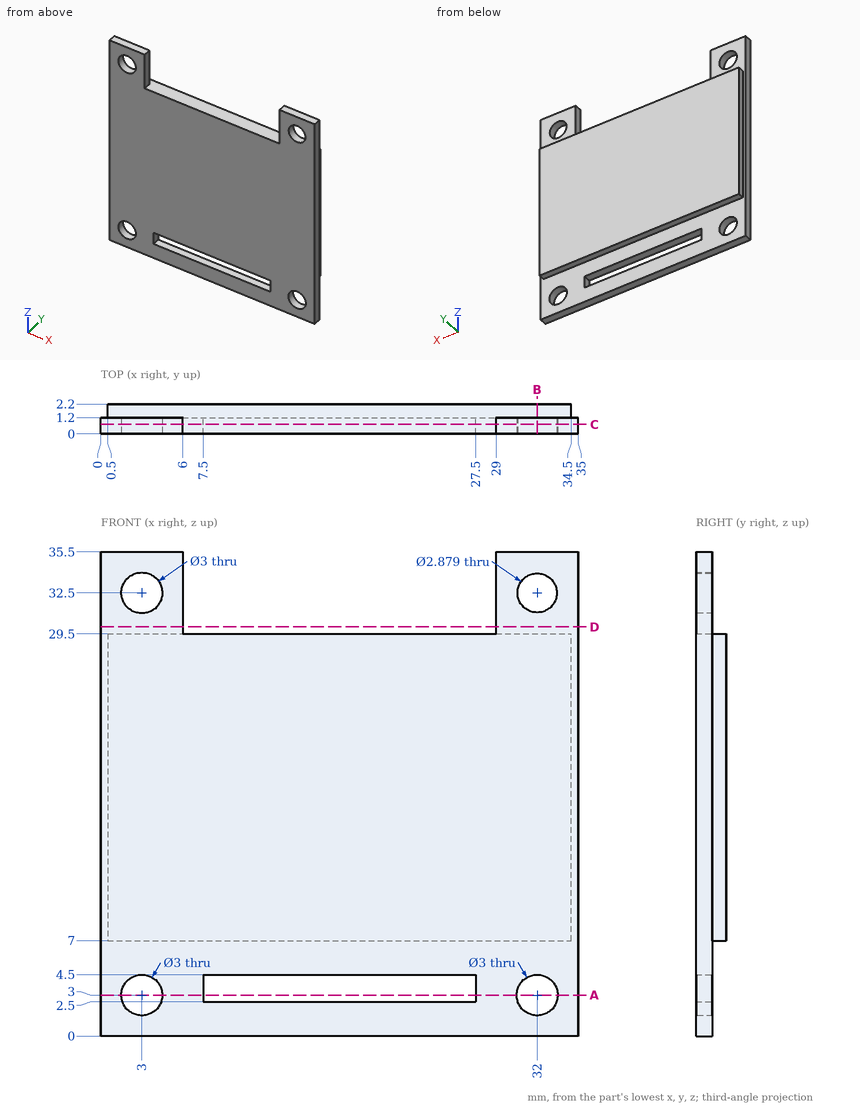
Check sheet for the drawn part. Datum: minimum x, y, z corner. Units: mm. Give positions to 0.01 mm unless a question says otherwise; leave off trailing zeros. Write each loop counter-clockwise with the first axis right and the second up, starting at its lowest first coordinate (ties: lowest second). Pieces come first, ordered by that corner, then holes. Notation, with made-up numbers: (79.5, -22) -> (85.5, -22) arc R36 ccw to (85.5, 12) -> close; hole circle Ø10 at (-39, 81.5). An arc over 180 degrees is marked (long way). Use one line per item in the form item = value. Start each with the question number.
1. Go/stop test with flat-tipped pins: P1, Ø0.8, axis at x = 20, y = 2, coming from the -Z side; P2, Ø1, axis at x = 13.5, y = 0.5, coming from the -Z side; P3, Ø3.5, axis at x = 3, z = 32.5, coming from the +Y side; P4, Ø2.5, axis at x = 32, z = 32.5, coming from the -Y side. Record where each tip stops, or that it passes through.
2. Section check D-D (z = 30). Record the cut outline in (x, y), and give its area (3 significant figures).
3. Section check C-C (y = 0.7). Record the cut outline in (x, z).
4. Section check B-B (x = 32). Record the cut outline in (y, z).
5. Section check A-A (z = 3). Record the cut outline in (x, y), and give its area (3 significant figures).
6. Thickness scan on line 1 along X through (y, z) = (0.7, 32.5); line 2 along X through (y, z) = (0.65, 3); line 3 along Z through (x, y) = (31, 0.9) (1 decimal). Record the ranges inside material, lowest first. Write a range as from..to.
Conclusion:
q1.P1 = 7
q1.P2 = 0
q1.P3 = 1.2
q1.P4 = through
q2.outline = (0, 0) -> (6, 0) -> (6, 1.2) -> (0, 1.2) -> close; (29, 0) -> (35, 0) -> (35, 1.2) -> (29, 1.2) -> close
q2.area = 14.4 mm²
q3.outline = (0, 0) -> (35, 0) -> (35, 35.5) -> (29, 35.5) -> (29, 29.5) -> (6, 29.5) -> (6, 35.5) -> (0, 35.5) -> close; hole circle Ø3 at (3, 3); hole circle Ø3 at (3, 32.5); hole (7.5, 2.5) -> (27.5, 2.5) -> (27.5, 4.5) -> (7.5, 4.5) -> close; hole circle Ø3 at (32, 3); hole circle Ø2.88 at (32, 32.5)
q4.outline = (0, 0) -> (1.2, 0) -> (1.2, 1.5) -> (0, 1.5) -> close; (0, 4.5) -> (1.2, 4.5) -> (1.2, 7) -> (2.2, 7) -> (2.2, 29.5) -> (1.2, 29.5) -> (1.2, 31.06) -> (0, 31.06) -> close; (0, 33.94) -> (1.2, 33.94) -> (1.2, 35.5) -> (0, 35.5) -> close
q5.outline = (0, 0) -> (1.5, 0) -> (1.5, 1.2) -> (0, 1.2) -> close; (4.5, 0) -> (7.5, 0) -> (7.5, 1.2) -> (4.5, 1.2) -> close; (27.5, 0) -> (30.5, 0) -> (30.5, 1.2) -> (27.5, 1.2) -> close; (33.5, 0) -> (35, 0) -> (35, 1.2) -> (33.5, 1.2) -> close
q5.area = 10.8 mm²
q6.line_1 = 0..1.5, 4.5..6, 29..30.56, 33.44..35
q6.line_2 = 0..1.5, 4.5..7.5, 27.5..30.5, 33.5..35
q6.line_3 = 0..1.9, 4.1..31.5, 33.5..35.5
